The listing builds one solid part. Answer for the finished solid, in the listing's coordinates (mm). A direction names the side the tool comes from. Round coordinates to 2 decimals unless told otherwise and drop trailing zeros. Write each loop counter-clockwise with the first axis right and the second up, starting at its lowest first coordinate (ties: lowest second). Pieces come first, ordered by that corner, then holes.
from build123d import *

# Parameters (mm, degrees)
F0_W     = 121.5
F0_H     = 30.5
F0_W_2   = 119.5
F0_H_2   = 28.5
F1_DEPTH = 155
F2_DEPTH = 1
F3_R     = 0.99999
F5_DEPTH = 30.5


# Not quite as in the source:
# - a fillet or chamfer is up to 0.001 mm smaller than in the source, because OpenCascade refuses the exact size


with BuildPart() as f1:
    # F0 (on Top) → F1 (new body)
    with BuildSketch(Plane.XY):
        with Locations((7.2500004172, -0.2499995828)):
            Rectangle(F0_W, F0_H)
        with Locations((7.2500004172, -0.2499995828)):
            Rectangle(F0_W_2, F0_H_2, mode=Mode.SUBTRACT)
    extrude(amount=F1_DEPTH)

    # F0 (on Top) → F2 (join)
    with BuildSketch(Plane.XY):
        with Locations((7.2500004172, -0.2499995828)):
            Rectangle(F0_W_2, F0_H_2)
    extrude(amount=F2_DEPTH)

    # F3 (radius 1 in the source; OpenCascade refuses exactly that, so slightly less here)
    f3_edges = [f1.edges().sort_by_distance(p)[0] for p in [
        (68, -15.5, 77.5),
        (68, 15, 77.5),
        (68, -0.25, 0),
        (7.25, 15, 0),
        (7.25, -15.5, 0),
        (-53.5, -0.25, 0),
        (-53.5, -15.5, 77.5),
        (-53.5, 15, 77.5),
        (7.25, -15.5, 155),
        (-53.5, -0.25, 155),
        (7.25, 15, 155),
        (68, -0.25, 155),
    ]]
    fillet(f3_edges, radius=F3_R)

    # F4 (on face) → F5 (cut, through all)
    with BuildSketch(Plane(origin=(0, 15.0000004172, 0), x_dir=(-1, 0, 0), z_dir=(0, 1, 0))):
        with BuildLine():
            ThreePointArc((26.5693810998, 154.00001), (27.8320116519, 159.3416659555), (28.2562680656, 164.8140996695))
            ThreePointArc((28.2562680656, 164.8140996695), (-12.7224341312, 199.8961117386), (-41.0693819342, 154.00001))
            Line((-41.0693819342, 154.00001), (-7.2500004172, 154.00001))
            Line((-7.2500004172, 154.00001), (26.5693810998, 154.00001))
        make_face()
        with BuildLine():
            Line((-7.2500004172, 154.00001), (-41.0693819342, 154.00001))
            ThreePointArc((-41.0693819342, 154.00001), (-7.2500004172, 129.3078311867), (26.5693810998, 154.00001))
            Line((26.5693810998, 154.00001), (-7.2500004172, 154.00001))
        make_face()
    extrude(amount=-F5_DEPTH, mode=Mode.SUBTRACT)


solid = f1.part
1. Section A-A on z = 87 is taken. Determine the outline of the cut face in (x, y), plus the area to 3 significant figures.
Geometry says:
outline: (-53.5, -14.5) arc R1 ccw to (-52.5, -15.5) - (67, -15.5) arc R1 ccw to (68, -14.5) - (68, 14) arc R1 ccw to (67, 15) - (-52.5, 15) arc R1 ccw to (-53.5, 14) - close; hole (-52.5, -14.5) - (67, -14.5) - (67, 14) - (-52.5, 14) - close
area: 299 mm2
2. Straight lines are drawn through the part: line 1 along X through (y, z) = (-6, 71); line 2 along Y through (x, z) = (-20, 73); line 3 along Z through (x, y) = (-20.5, 6). For each, find the intervals that lie inside material, in ascending order.
Geometry says:
line 1: x = -53.5 to -52.5, 67 to 68
line 2: y = -15.5 to -14.5, 14 to 15
line 3: z = 0 to 1
3. For a pull along Z with two mould halves and no side action, classify faces 3 (the face through (6, 0, 0)), 4 (the face through (6, 15, 76)), 5 (the face through (6, 0, 1)) as released by +Z, released by -Z, zero draft, split by the parting line, or undercut.
Geometry says:
face 3: released by -Z
face 4: zero draft
face 5: released by +Z
4. Section D-D on x = 27 is taken. Determine the outline of the cut face in (y, z), plus the area to 3 significant figures.
Geometry says:
outline: (-15.5, 1) arc R1 ccw to (-14.5, 0) - (14, 0) arc R1 ccw to (15, 1) - (15, 135.31) - (14, 135.31) - (14, 1) - (-14.5, 1) - (-14.5, 135.31) - (-15.5, 135.31) - close
area: 299 mm2
5. Given pin 1 (14 mm diameter, centred on x = -15.5, y = 6.5, fed in from +Z), flat-ended and moving along its own axis, determine where the tip first touches the part or whether it passes through.
Geometry says:
pin 1: stops at z = 1
6. A tool of negligible diameter and unlimited length cuts with its end or side. For faces 1 (the face through (-53.5, 0, 76)), 2 (the face through (6, -14.5, 77)), from which of +Z, -Z, +X, -X, +Y, -Y can it reach the whole face along a straight path? Write none if from no direction.
Geometry says:
face 1: +Z, -Z, -X, +Y, -Y
face 2: +Z
